from build123d import *

# Parameters (mm, degrees)
SKETCH1_W           = 55
SKETCH1_H           = 48
SKETCH1_R           = 3
BOSS_EXTRUDE1_DEPTH = 8
SKETCH2_W           = 55
SKETCH2_H           = 27
BOSS_EXTRUDE2_DEPTH = 6
SKETCH3_W           = 15
SKETCH3_H           = 35
BOSS_EXTRUDE3_DEPTH = 2.5
FILLET1_R           = 2
RIB1_REACH          = 75.091
SKETCH4_WALL_W      = 185.181394164
SKETCH4_WALL_H      = 5
BOSS_EXTRUDE5_REACH = 77.566
BOSS_EXTRUDE6_DEPTH = 35
FILLET3_R           = 35
FILLET4_R           = 32
FILLET5_R           = 35
FILLET6_R           = 3


with BuildPart() as part:
    # Sketch1 → Boss-Extrude1 (new body)
    with BuildSketch(Plane.XY):
        Rectangle(SKETCH1_W, SKETCH1_H)
        with Locations((20, 0.5)):
            Circle(SKETCH1_R, mode=Mode.SUBTRACT)
        with Locations((-20, 0.5)):
            Circle(SKETCH1_R, mode=Mode.SUBTRACT)
    extrude(amount=BOSS_EXTRUDE1_DEPTH)

    # Sketch2 → Boss-Extrude2 (add)
    with BuildSketch(Plane(origin=(0, 24, 0), x_dir=(1, 0, 0), z_dir=(0, 1, 0))):
        with Locations((0, 5.5)):
            Rectangle(SKETCH2_W, SKETCH2_H)
    extrude(amount=BOSS_EXTRUDE2_DEPTH)

    # Sketch3 → Boss-Extrude3 (add, symmetric)
    with BuildSketch(Plane(origin=(0, 0, 0), x_dir=(0, 0, -1), z_dir=(1, 0, 0))):
        with Locations((11.5, 47.5)):
            Rectangle(SKETCH3_W, SKETCH3_H)
    extrude(amount=BOSS_EXTRUDE3_DEPTH, both=True)

    # Fillet1
    fillet1_edges = [part.edges().sort_by_distance(p)[0] for p in [
        (0, 24, 0),
    ]]
    fillet(fillet1_edges, radius=FILLET1_R)

    # Sketch4 wall → Rib1 (add, up to next)
    with BuildSketch(Plane(origin=(0, 47.5, 2), x_dir=(0, -0.945945945946, 0.324324324324), z_dir=(0, -0.324324324324, -0.945945945946)), mode=Mode.PRIVATE) as rib1_sk1:
        Rectangle(SKETCH4_WALL_W, SKETCH4_WALL_H)
    rib1_tool1 = extrude(rib1_sk1.sketch, amount=RIB1_REACH, mode=Mode.PRIVATE) - part.part
    add(rib1_tool1.solids().sort_by_distance((0, 47.5, 2))[0])

    # Boss-Extrude5: up to this plane
    boss_extrude5_end = Plane(origin=(0, 65, -4), z_dir=(0, 0.3243243243243244, 0.945945945945946))
    # Sketch5 → Boss-Extrude5 (add, up to the surface)
    with BuildSketch(Plane(origin=(0, 0, -19), x_dir=(-1, 0, 0), z_dir=(0, 0, -1)), mode=Mode.PRIVATE) as boss_extrude5_sk1:
        Polygon((-27.5, 30), (-2.5, 65), (-2.5, 30), align=None)
    boss_extrude5_tool1 = split(extrude(boss_extrude5_sk1.sketch, amount=-BOSS_EXTRUDE5_REACH, mode=Mode.PRIVATE), bisect_by=boss_extrude5_end, keep=Keep.BOTH, mode=Mode.PRIVATE)
    boss_extrude5 = boss_extrude5_tool1.solids().sort_by_distance((10.833333, 41.666667, -19))[0]
    add(boss_extrude5)

    # Mirror1: Boss-Extrude5 across plane
    add(boss_extrude5.mirror(Plane(origin=(0, 0, 0), x_dir=(0, 0, 1), z_dir=(1, 0, 0))))

    # Sketch7 → Boss-Extrude6 (add)
    with BuildSketch(Plane(origin=(0, 65, 0), x_dir=(1, 0, 0), z_dir=(0, 1, 0))):
        Polygon((2.5, 19), (-2.5, 19), (98, 119.5), (152.5, 119.5), (152.5, 116), (99.5, 116), align=None)
    extrude(amount=-BOSS_EXTRUDE6_DEPTH)

    # Fillet3
    fillet3_edges = [part.edges().sort_by_distance(p)[0] for p in [
        (98, 47.5, -119.5),
    ]]
    fillet(fillet3_edges, radius=FILLET3_R)

    # Fillet4
    fillet4_edges = [part.edges().sort_by_distance(p)[0] for p in [
        (99.5, 47.5, -116),
    ]]
    fillet(fillet4_edges, radius=FILLET4_R)

    # Fillet5
    fillet5_edges = [part.edges().sort_by_distance(p)[0] for p in [
        (-2.5, 47.5, -19),
    ]]
    fillet(fillet5_edges, radius=FILLET5_R)

    # Fillet6
    # the kernel refuses this fillet: 3 mm, written as the material it adds along each edge
    with BuildSketch(Plane(origin=(2.5, 65, -19), x_dir=(1, 0, 0), z_dir=(0, -1, 0))) as fillet6_piece_1_section:
        with BuildLine():
            CenterArc((FILLET6_R * 2.41421356237, -FILLET6_R), FILLET6_R, 90, 135)
            Line((FILLET6_R * 1.70710678119, -FILLET6_R * 1.70710678119), (0, 0))
            Line((0, 0), (FILLET6_R * 2.41421356237, 0))
        make_face()
    fillet6_piece_1 = extrude(amount=35, mode=Mode.PRIVATE)
    fillet6_piece_1 = split(fillet6_piece_1, bisect_by=Plane(origin=(12.87170443, 50.479613798, -20.318339623), z_dir=(-0.813733471206735, -0.5812381937190964, 0)), keep=Keep.TOP, mode=Mode.PRIVATE)
    add(fillet6_piece_1)


solid = part.part
Could you check a few things on this model? Use its own coordinates, in mm. A direction names the side the tool comes from. Coordinates: 2 decimals unless noted, no trailing zeros. Order: outer loops, then holes, each group sorted by start corner. A loop starts at its lowest first (then second) coordinate and runs counter-clockwise, first axis right, second up.
Q1. Will these pins go through, and if not, where does the flat tip stop? pin 1 (8 mm diameter, centred on x = -20, y = 0.5, fed in from -Z); pin 2 (9.5 mm diameter, centred on x = -13.5, y = 40.5, fed in from -Z); pin 3 (18.5 mm diameter, centred on x = -5, z = -12, fed in from -Y).
Q2. Suppose I cut it at D-D on z = -42. Please give me the cut outline in (x, y), and give its area (3 significant figures).
Q3. Thinking about a two-plate mould opening in X: for faces 5 (the cylindrical face through (6.99, 44.78, -20.81)), 6 (the flat face through (0, 24, -11)), 7 (the cylindrical face through (17, 0.6, 3.9)), which applies, released by +X, released by -X, zero draft, split by the parting line, or undercut?
Q4. Suppose I cut it at A-A on x = 20. Please give me the cut outline in (y, z), and give its area (3 significant figures).
Q5. Which directions (+Z, -Z, +X, -X, +Y, -Y) give clear straight access to the entire face, cutting with the end or side of a thin tool? Please do faces 1 (the flat face through (68, 30, -88)), 2 (the flat face through (0, 29, -19)), 3 (the flat face through (0, 3, 8)), 4 (the flat face through (14.83, 47.74, -7.84)).
Q6. Suppose I cut it at B-B on y = 0.5. Please give me the cut outline in (x, z), and give its area (3 significant figures).
Q7. Please list where these lines run through material, in increasing order: L1, parallel to X at y = 0, z = 3; L2, parallel to Z at x = -17, y = 1; L3, parallel to Y at x = 20, z = 2.25.
Q8. Suppose I cut it at C-C on x = -20. Please give me the cut outline in (y, z).
Answer:
1. pin 1: stops at z = 0
1. pin 2: stops at z = -19.99
1. pin 3: stops at y = 24
2. outline: (20.5, 30) - (25.5, 30) - (25.5, 65) - (20.5, 65) - close
2. area: 175 mm2
3. face 5: released by +X
3. face 6: zero draft
3. face 7: undercut
4. outline: (-24, 0) - (-2.5, 0) - (-2.5, 8) - (-24, 8) - close; (3.5, 0) - (22, 0) arc R2 cw to (24, -2) - (24, -19) - (40.5, -19) - (40.5, 4.4) - (30, 8) - (3.5, 8) - close; (30, -41.5) - (65, -41.5) - (65, -36.5) - (30, -36.5) - close
4. area: 938 mm2
5. face 1: -Z, +X, -X, -Y
5. face 2: -Y
5. face 3: +Z, +X, -X, +Y, -Y
5. face 4: +Z, +X, +Y
6. outline: (-27.5, 0) - (-23, 0) - (-23, 8) - (-27.5, 8) - close; (-17, 0) - (17, 0) - (17, 8) - (-17, 8) - close; (23, 0) - (27.5, 0) - (27.5, 8) - (23, 8) - close
6. area: 344 mm2
7. L1: x = -27.5 to -22.96, -17.04 to 17.04, 22.96 to 27.5
7. L2: z = 0 to 8
7. L3: y = -24 to -2.5, 3.5 to 40.5
8. outline: (-24, 0) - (-2.5, 0) - (-2.5, 8) - (-24, 8) - close; (3.5, 0) - (22, 0) arc R2 cw to (24, -2) - (24, -19) - (40.5, -19) - (40.5, 4.4) - (30, 8) - (3.5, 8) - close
